Geometry: final body of the model. Coordinates: model frame, mm. Round coordinates to 2 decimals unless told otherwise and drop trailing zeros. Order: outer loops, then holes, each group sorted by start corner. A loop starts at its lowest first (then second) coordinate and runs counter-clockwise, first axis right, second up. Notation, with made-up numbers: M -15.5,25.25 L 10.5,25.25 A22 cw 10.5,39.25 Z; hole C 36.25,9 d1. An arc over 180 degrees is marked long. Return JSON: item names as keys, results as strings. Group by question number.
Q1. Cut plane A-A on y = 101.6. Output: boundary loops of the cut face in (x, z).
Q2. Cut plane C-C on x = 11.5. Output: boundary loops of the cut face in (y, z), and give its area (3 significant figures).
Q3. Mould query, pull axis X, two halves, no side actions, for faces 1 (the face through (20.56, 98.51, 2.32)), 2 (the face through (19.228, 0.833, 2.317)), 3 (the face through (33.02, 86, 2)). Classes: released by +X, released by -X, zero draft, split by the parting line, or undercut.
Q4. Contact query for flat-ended pins moving along their axis: pin 1 (1.5 mm diameter, centred on x = 29.5, z = 4, fed in from -Y); pin 2 (1.5 mm diameter, centred on x = 20.5, y = 87, fed in from -Z). Output: stop coordinate, or through.
Q5. Cut plane B-B on z = 0.95. Output: boundary loops of the cut face in (x, y) (1 decimal).
Q6. Ray query, probe 1 along Y at (x, z) = (28.5, 4.1); probe 2 along Y at (x, z) = (23.5, 4); probe 3 along Y at (x, z) = (14, 3.45). Return the intervals inside material, ascending.
```python
from build123d import *

# Parameters (mm, degrees)
F0_R        = 5.08
F1_DEPTH    = 4.699
F2_T1_DEPTH = 25.7410489686
F2_T3_DEPTH = 55.499


# Not quite as in the source:
# - a fillet or chamfer that OpenCascade refuses, or shapes differently, is made with other operations: its cross-section is extruded or revolved along the edge and cut away or added
# - a feature names something its author has since deleted; it is built from what else it names


with BuildPart() as f1:
    # F0 (on Top) → F1 (new body)
    with BuildSketch(Plane.XY):
        with BuildLine():
            Line((31.4325, 165.1), (1.5875, 165.1))
            ThreePointArc((1.5875, 165.1), (1.1225320151, 163.9774679849), (0, 163.5125))
            Line((0, 163.5125), (0, 19.05))
            Line((0, 19.05), (19.05, 0))
            Line((19.05, 0), (33.02, 0))
            Line((33.02, 0), (33.02, 163.5125))
            ThreePointArc((33.02, 163.5125), (31.8974679849, 163.9774679849), (31.4325, 165.1))
        make_face()
        with Locations((25.2715107054, 10.16)):
            Circle(F0_R, mode=Mode.SUBTRACT)
        with Locations((24.5934482664, 101.6)):
            Circle(F0_R, mode=Mode.SUBTRACT)
    extrude(amount=F1_DEPTH)

    # F2: fillet of radius 10.16 on 3 edges, made by hand

    # F2_s2 → F2_t1 (cut)
    with BuildSketch(Plane.XY.offset(-10.5210244843)):
        with BuildLine():
            ThreePointArc((0, 23.2584097937), (0.7733839497, 19.3703461209), (2.9757951031, 16.0742048969))
            Line((2.9757951031, 16.0742048969), (0, 19.05))
            Line((0, 19.05), (0, 23.2584097937))
        make_face()
        with BuildLine():
            ThreePointArc((16.0742048969, 2.9757951031), (19.3703461209, 0.7733839497), (23.2584097937, 0))
            Line((23.2584097937, 0), (19.05, 0))
            Line((19.05, 0), (16.0742048969, 2.9757951031))
        make_face()
    extrude(amount=F2_T1_DEPTH, mode=Mode.SUBTRACT)

    # F2_s4 → F2_t3 (cut)
    with BuildSketch(Plane.XY.offset(-25.4)):
        with BuildLine():
            ThreePointArc((22.86, 0), (30.0442048969, 2.9757951031), (33.02, 10.16))
            Line((33.02, 10.16), (33.02, 0))
            Line((33.02, 0), (22.86, 0))
        make_face()
    extrude(amount=F2_T3_DEPTH, mode=Mode.SUBTRACT)


solid = f1.part
```
Result sheet:
{
 "1": {"outline": "M 0,0 L 19.51,0 L 19.51,4.7 L 0,4.7 Z; M 29.67,0 L 33.02,0 L 33.02,4.7 L 29.67,4.7 Z"},
 "2": {"outline": "M 7.55,0 L 165.1,0 L 165.1,4.7 L 7.55,4.7 Z", "area": "740 mm²"},
 "3": {"face 1": "undercut", "face 2": "released by -X", "face 3": "released by +X"},
 "4": {"pin 1": "stops at y = 1.88", "pin 2": "stops at z = 0"},
 "5": {"outline": "M 0,23.3 A10.2 ccw 3,16.1 L 16.1,3 A10.2 ccw 23.1,0 A10.2 ccw 33,10.2 L 33,163.5 A1.6 cw 31.4,165.1 L 1.6,165.1 A1.6 cw 0,163.5 Z; hole C 24.6,101.6 d10.2; hole C 25.3,10.2 d10.2"},
 "6": {"probe 1": "y = 1.71 to 6.24, 14.08 to 98.35, 104.85 to 165.1", "probe 2": "y = 0.02 to 5.4, 14.92 to 96.64, 106.56 to 165.1", "probe 3": "y = 5.05 to 165.1"}
}
